from build123d import *

# Parameters (mm, degrees)
P_IDAT_VYSUNUT_M2_DEPTH  = 2.5
SKICA3_W                 = 0.8
SKICA3_H                 = 0.8
ODEBRAT_VYSUNUT_M1_DEPTH = 2.5


# Read off the part's stored shape, not the designer's step: Přidat vysunutím2
with BuildPart() as part:
    # Přidat vysunutím2 outline → Přidat vysunutím2 (new body)
    with BuildSketch(Plane.XY):
        with BuildLine():
            Line((2.40336004, -19.590083306), (2.40336004, -16.441317707))
            ThreePointArc((2.40336004, -16.441317707), (1.30336004, -15.341317707), (0.20336004, -16.441317707))
            Line((0.20336004, -16.441317707), (-0.14663996, -16.441317707))
            ThreePointArc((-0.14663996, -16.441317707), (-1.24602276, -15.34131788), (-2.346639267, -16.440083307))
            Line((-2.346639267, -16.440083307), (-2.696640653, -16.440083307))
            ThreePointArc((-2.696640653, -16.440083307), (-3.79725716, -15.34131788), (-4.89663996, -16.441317707))
            Line((-4.89663996, -16.441317707), (-5.24663996, -16.441317707))
            ThreePointArc((-5.24663996, -16.441317707), (-6.34663996, -15.341317707), (-7.44663996, -16.441317707))
            Line((-7.44663996, -16.441317707), (-7.79663996, -16.441317707))
            Line((-7.79663996, -16.441317707), (-7.79663996, -16.399925636))
            ThreePointArc((-7.79663996, -16.399925636), (-8.89663996, -15.299925636), (-9.99663996, -16.399925636))
            Line((-9.99663996, -16.399925636), (-9.99663996, -16.441317707))
            Line((-9.99663996, -16.441317707), (-10.34663996, -16.441317707))
            ThreePointArc((-10.34663996, -16.441317707), (-11.44663996, -15.341317707), (-12.54663996, -16.441317707))
            Line((-12.54663996, -16.441317707), (-12.89663996, -16.441317707))
            ThreePointArc((-12.89663996, -16.441317707), (-13.99663996, -15.341317707), (-15.09663996, -16.441317707))
            Line((-15.09663996, -16.441317707), (-15.09663996, -19.590083306))
            ThreePointArc((-15.09663996, -19.590083306), (-13.99663996, -20.690083306), (-12.89663996, -19.590083306))
            Line((-12.89663996, -19.590083306), (-12.54663996, -19.590083306))
            ThreePointArc((-12.54663996, -19.590083306), (-11.44663996, -20.690083306), (-10.34663996, -19.590083306))
            Line((-10.34663996, -19.590083306), (-9.99663996, -19.590083306))
            Line((-9.99663996, -19.590083306), (-9.99663996, -19.631475378))
            ThreePointArc((-9.99663996, -19.631475378), (-8.89663996, -20.731475378), (-7.79663996, -19.631475378))
            Line((-7.79663996, -19.631475378), (-7.79663996, -19.590083306))
            Line((-7.79663996, -19.590083306), (-7.44663996, -19.590083306))
            ThreePointArc((-7.44663996, -19.590083306), (-6.34663996, -20.690083306), (-5.24663996, -19.590083306))
            Line((-5.24663996, -19.590083306), (-4.89663996, -19.590083306))
            ThreePointArc((-4.89663996, -19.590083306), (-3.79663996, -20.690083306), (-2.69663996, -19.590083306))
            Line((-2.69663996, -19.590083306), (-2.34663996, -19.590083306))
            ThreePointArc((-2.34663996, -19.590083306), (-1.24663996, -20.690083306), (-0.14663996, -19.590083306))
            Line((-0.14663996, -19.590083306), (0.20336004, -19.590083306))
            ThreePointArc((0.20336004, -19.590083306), (1.30336004, -20.690083306), (2.40336004, -19.590083306))
        make_face()
    extrude(amount=P_IDAT_VYSUNUT_M2_DEPTH)

    # Skica3 → Odebrat vysunutím1 (cut)
    with BuildSketch(Plane.XY.offset(2.5)):
        with Locations((-13.99663996, -16.715700507)):
            Rectangle(SKICA3_W, SKICA3_H)
        with Locations((-13.99663996, -19.315700507)):
            Rectangle(SKICA3_W, SKICA3_H)
        with Locations((-8.89663996, -16.715700507)):
            Rectangle(SKICA3_W, SKICA3_H)
        with Locations((-11.44663996, -16.715700507)):
            Rectangle(SKICA3_W, SKICA3_H)
        with Locations((-11.44663996, -19.315700507)):
            Rectangle(SKICA3_W, SKICA3_H)
        with Locations((-8.89663996, -19.315700507)):
            Rectangle(SKICA3_W, SKICA3_H)
        with Locations((-6.34663996, -16.715700507)):
            Rectangle(SKICA3_W, SKICA3_H)
        with Locations((-6.34663996, -19.315700507)):
            Rectangle(SKICA3_W, SKICA3_H)
        with Locations((-3.79663996, -16.715700507)):
            Rectangle(SKICA3_W, SKICA3_H)
        with Locations((-3.79663996, -19.315700507)):
            Rectangle(SKICA3_W, SKICA3_H)
        with Locations((-1.24663996, -16.715700507)):
            Rectangle(SKICA3_W, SKICA3_H)
        with Locations((-1.24663996, -19.315700507)):
            Rectangle(SKICA3_W, SKICA3_H)
        with Locations((1.30336004, -16.715700507)):
            Rectangle(SKICA3_W, SKICA3_H)
        with Locations((1.30336004, -19.315700507)):
            Rectangle(SKICA3_W, SKICA3_H)
    extrude(amount=-ODEBRAT_VYSUNUT_M1_DEPTH, mode=Mode.SUBTRACT)


solid = part.part
The listing builds one solid part. Answer for the finished solid, in the listing's coordinates (mm). A direction names the side the tool comes from. Coordinates: 2 decimals unless noted, no trailing zeros. Loops run counter-clockwise (first coordinate to the right, second up) from the corner with the lowest first, then second, coordinate; pieces in that order, holes last. Notation, with made-up numbers: (7, 46.5) -> (41, 46.5) arc R24 ccw to (41, 77.5) -> close; hole circle Ø10 at (-20, 81). An arc over 180 degrees is marked (long way). Write item = value, one per line. Start each with the question number.
1) Straight lines are drawn through the part: line 1 (Y direction, x = -14, z = 1.85); line 2 (Y direction, x = -13.75, z = 2.35); line 3 (Y direction, x = -7.5, z = 1.25). For each, find the intervals that lie inside material, in ascending order. Write a range as from..to.
2) A cutting plane is placed at D-D (x = -11.5). Give the vertices of the cut face in (y, z), then the cut area to 3 significant figures.
3) The mould has two halves that part along Y. Classify faces 1 (the face through (-11.5, -18.916, 1.3)), 2 (the face through (-11.47, -20.69, 1.23)), 3 (the face through (2.403, -18, 1)): released by +Y, released by -Y, zero draft, split by the parting line, or undercut.
4) A cutting plane is placed at A-A (y = -19.2). Count the separate pieces of the cut face and the enclosed holes in it, then the cut area to 4 significant figures.
5) Given pin 1 Ø0.9 at (x, z) = (1, 1) entering from +Y; pin 2 Ø0.6 at (x, z) = (-1.5, 1) entering from -Y, each flat-ended and moving along its own axis, determine where each tip first touches the part or whether it passes through.
6) A cutting plane is placed at C-C (y = -15.9). Give the vertices of the cut face in (x, z), then the cut area to 3 significant figures.
7) A tool of negligible diameter and unlimited length cuts with its end or side. For faces 4 (the face through (-6, -18, 2.5)), 5 (the face through (-9, -19.716, 1)), from which of +Z, -Z, +X, -X, +Y, -Y can it reach the whole face along a straight path? Write none if from no direction.
8) A cutting plane is placed at B-B (x = -13.75). Give the vertices of the cut face in (y, z).
Responses:
q1.line_1 = -20.69..-19.72, -18.92..-17.12, -16.32..-15.34
q1.line_2 = -20.66..-19.72, -18.92..-17.12, -16.32..-15.37
q1.line_3 = -19.59..-16.44
q2.outline = (-20.69, 0) -> (-19.72, 0) -> (-19.72, 2.5) -> (-20.69, 2.5) -> close; (-18.92, 0) -> (-17.12, 0) -> (-17.12, 2.5) -> (-18.92, 2.5) -> close; (-16.32, 0) -> (-15.34, 0) -> (-15.34, 2.5) -> (-16.32, 2.5) -> close
q2.area = 9.37 mm²
q3.face_1 = undercut
q3.face_2 = released by -Y
q3.face_3 = zero draft
q4.separate_pieces = 8
q4.enclosed_holes = 0
q4.area = 29.75 mm²
q5.pin_1 = -15.34
q5.pin_2 = -20.69
q6.outline = (-14.95, 0) -> (-13.04, 0) -> (-13.04, 2.5) -> (-14.95, 2.5) -> close; (-12.4, 0) -> (-10.49, 0) -> (-10.49, 2.5) -> (-12.4, 2.5) -> close; (-9.88, 0) -> (-7.92, 0) -> (-7.92, 2.5) -> (-9.88, 2.5) -> close; (-7.3, 0) -> (-5.39, 0) -> (-5.39, 2.5) -> (-7.3, 2.5) -> close; (-4.75, 0) -> (-2.84, 0) -> (-2.84, 2.5) -> (-4.75, 2.5) -> close; (-2.2, 0) -> (-0.29, 0) -> (-0.29, 2.5) -> (-2.2, 2.5) -> close; (0.35, 0) -> (2.26, 0) -> (2.26, 2.5) -> (0.35, 2.5) -> close
q6.area = 33.6 mm²
q7.face_4 = +Z, +X, -X, +Y, -Y
q7.face_5 = +Z, -Z
q8.outline = (-20.66, 0) -> (-19.72, 0) -> (-19.72, 2.5) -> (-20.66, 2.5) -> close; (-18.92, 0) -> (-17.12, 0) -> (-17.12, 2.5) -> (-18.92, 2.5) -> close; (-16.32, 0) -> (-15.37, 0) -> (-15.37, 2.5) -> (-16.32, 2.5) -> close
